```python
from build123d import *

# Parameters (mm, degrees)
ESBO_O2_W                                   = 14
ESBO_O2_H                                   = 46
RESSALTO_EXTRUS_O1_DEPTH                    = 6
CORTE_EXTRUS_O1_DEPTH                       = 49.456165758
FURO_DE_DI_METRO_7_5_7_5_1_D                = 7.5
CORTE_EXTRUS_O2_DEPTH                       = 49.456165758
ESBO_O10_W                                  = 5
ESBO_O10_H                                  = 4
RESSALTO_EXTRUS_O2_DEPTH                    = 5
BROCA_DE_ROSQUEAR_PARA_TARRAXA_DE_M31_D     = 2.5
BROCA_DE_ROSQUEAR_PARA_TARRAXA_DE_M31_DEPTH = 4
BROCA_DE_ROSQUEAR_PARA_TARRAXA_DE_M31_TIP   = 0.751075774
FURO_DE_DI_METRO_6_0_6_1_D                  = 6
CHANFRO1_SIZE                               = 1
FURO_DE_DI_METRO_3_0_3_1_D                  = 3
FURO_DE_DI_METRO_3_0_3_1_DEPTH              = 1
FURO_DE_DI_METRO_3_0_3_1_TIP                = 0.901290929
ESBO_O14_R                                  = 5.55
CORTE_EXTRUS_O4_DEPTH                       = 5


with BuildPart() as part:
    # Esboço2 → Ressalto-extrusão1 (new body)
    with BuildSketch(Plane(origin=(0, 0, 0), x_dir=(1, 0, 0), z_dir=(0, 1, 0))):
        with Locations((7, 23)):
            Rectangle(ESBO_O2_W, ESBO_O2_H)
    extrude(amount=RESSALTO_EXTRUS_O1_DEPTH)

    # Esboço6 → Corte-extrusão1 (cut, through all)
    with BuildSketch(Plane(origin=(0, 6, 0), x_dir=(1, 0, 0), z_dir=(0, 1, 0))):
        with BuildLine():
            Line((4.5, 46), (4.5, 31.538348415))
            ThreePointArc((4.5, 31.538348415), (1.233718703, 28.968626967), (0, 25))
            Line((0, 25), (0, 46))
            Line((0, 46), (4.5, 46))
        make_face()
        with BuildLine():
            Line((9.5, 46), (9.5, 31.538348415))
            ThreePointArc((9.5, 31.538348415), (12.766281297, 28.968626967), (14, 25))
            Line((14, 25), (14, 46))
            Line((14, 46), (9.5, 46))
        make_face()
    extrude(amount=-CORTE_EXTRUS_O1_DEPTH, mode=Mode.SUBTRACT)

    # Furo de diâmetro Ø7.5 (7.5)1 (through all)
    with Locations(Plane(origin=(7, 6, -13.5), x_dir=(0, 0, 1), z_dir=(0, 1, 0))):
        with Locations((0, 0)):
            Hole(FURO_DE_DI_METRO_7_5_7_5_1_D / 2)

    # Esboço9 → Corte-extrusão2 (cut, through all)
    with BuildSketch(Plane(origin=(0, 6, 0), x_dir=(1, 0, 0), z_dir=(0, 1, 0))):
        with BuildLine():
            Line((0, 13.5), (0, 0))
            Line((0, 0), (4.5, 0))
            Line((4.5, 0), (4.5, 6.961651585))
            ThreePointArc((4.5, 6.961651585), (1.233718703, 9.531373033), (0, 13.5))
        make_face()
        with BuildLine():
            Line((9.5, 0), (9.5, 6.961651585))
            ThreePointArc((9.5, 6.961651585), (12.766281297, 9.531373033), (14, 13.5))
            Line((14, 13.5), (14, 0))
            Line((14, 0), (9.5, 0))
        make_face()
    extrude(amount=-CORTE_EXTRUS_O2_DEPTH, mode=Mode.SUBTRACT)

    # Esboço10 → Ressalto-extrusão2 (add)
    with BuildSketch(Plane(origin=(0, 6, 0), x_dir=(1, 0, 0), z_dir=(0, 1, 0))):
        with Locations((7, 44)):
            Rectangle(ESBO_O10_W, ESBO_O10_H)
        with Locations((7, 2)):
            Rectangle(ESBO_O10_W, ESBO_O10_H)
    extrude(amount=RESSALTO_EXTRUS_O2_DEPTH)

    # Broca de rosquear para tarraxa de M31
    with Locations(Plane(origin=(7, 11, -2), x_dir=(0, 0, 1), z_dir=(0, 1, 0))):
        with Locations((0, 0), (-42, 0)):
            Hole(BROCA_DE_ROSQUEAR_PARA_TARRAXA_DE_M31_D / 2, depth=BROCA_DE_ROSQUEAR_PARA_TARRAXA_DE_M31_DEPTH)
            with Locations((0, 0, -(BROCA_DE_ROSQUEAR_PARA_TARRAXA_DE_M31_DEPTH + BROCA_DE_ROSQUEAR_PARA_TARRAXA_DE_M31_TIP / 2))):  # 118° drill point
                Cone(0, BROCA_DE_ROSQUEAR_PARA_TARRAXA_DE_M31_D / 2, BROCA_DE_ROSQUEAR_PARA_TARRAXA_DE_M31_TIP, mode=Mode.SUBTRACT)

    # Furo de diâmetro Ø6.0 (6)1 (through all)
    with Locations(Plane(origin=(7, 6, -25), x_dir=(0, 0, 1), z_dir=(0, 1, 0))):
        with Locations((0, 0)):
            Hole(FURO_DE_DI_METRO_6_0_6_1_D / 2)

    # Chanfro1
    chanfro1_edges = [part.edges().sort_by_distance(p)[0] for p in [
        (0, 0, -19.25),
        (7, 0, -46),
        (9.5, 5.5, -46),
        (12.766281297, 0, -28.968626967),
        (9.5, 0, -38.769174208),
        (4.5, 0, -38.769174208),
        (4.5, 5.5, -46),
        (1.233718703, 0, -28.968626967),
        (14, 0, -19.25),
        (7, 0, 0),
        (1.233718703, 0, -9.531373033),
        (4.5, 0, -3.480825792),
        (4.5, 5.5, 0),
        (9.5, 0, -3.480825792),
        (9.5, 5.5, 0),
        (12.766281297, 0, -9.531373033),
    ]]
    chamfer(chanfro1_edges, length=CHANFRO1_SIZE)

    # Furo de diâmetro Ø3.0 (3)1
    with Locations(Plane(origin=(7, 6, -36), x_dir=(0, 0, 1), z_dir=(0, 1, 0))):
        with Locations((0, 0)):
            Hole(FURO_DE_DI_METRO_3_0_3_1_D / 2, depth=FURO_DE_DI_METRO_3_0_3_1_DEPTH)
            with Locations((0, 0, -(FURO_DE_DI_METRO_3_0_3_1_DEPTH + FURO_DE_DI_METRO_3_0_3_1_TIP / 2))):  # 118° drill point
                Cone(0, FURO_DE_DI_METRO_3_0_3_1_D / 2, FURO_DE_DI_METRO_3_0_3_1_TIP, mode=Mode.SUBTRACT)

    # Esboço14 → Corte-extrusão4 (cut)
    with BuildSketch(Plane.XZ):
        with Locations(Location((7, -25, 0), (0, 0, 270))):
            Circle(ESBO_O14_R)
    extrude(amount=-CORTE_EXTRUS_O4_DEPTH, mode=Mode.SUBTRACT)


solid = part.part
```
The listing builds one solid part. Answer for the finished solid, in the listing's coordinates (mm). A direction names the side the tool comes from. Coordinates: 2 decimals unless noted, no trailing zeros. Loops run counter-clockwise (first coordinate to the right, second up) from the corner with the lowest first, then second, coordinate; pieces in that order, holes last. Notation, with made-up numbers: (56.5, 17) - (115.5, 17) arc R32 ccw to (115.5, 54) - close; hole circle Ø4 at (-3.75, 51). An arc over 180 degrees is marked (long way). Use a Markdown table: item, result. Add a question column.
1) For faces 1 (the flat face through (9.5, 5, -40)), 2 (the cylindrical face through (4.718, 2.958, -10.524)), 3 (the cylindrical face through (6.1, 5.5, -34.8)), 4 (the flat face through (5, 0.5, -38)), determine the directions among +Z, -Z, +X, -X, +Y, -Y from which every point of the face is accessible in a straight line to the end or side of a thin tool.
2) The part is cut by section B-B, the plane z = -41.5. Give the vertices of the cut face in (x, y), and give its area (3 significant figures).
3) Find the intervals of material crossed by line 1 (Z direction, x = 7, y = 9.5); line 2 (X direction, y = 8.75, z = -2); line 3 (Z direction, x = 9.75, y = 3.5), in increasing order.
4) Given pin 1 (5.5 mm diameter, centred on x = 8.5, z = -24, fed in from -Y); pin 2 (4 mm diameter, centred on x = 5, z = -22.5, fed in from +Y); pin 3 (3 mm diameter, centred on x = 2, y = 5.5, fed in from +Z); pin 4 (3.5 mm diameter, centred on x = 7, z = -25, fed in from -Y), each flat-ended and moving along its own axis, determine where each tip first touches the part or whether it passes through.
5) The mould has two halves that part along X. Classify faces 5 (the cylindrical face through (7.1, 5.5, -22)), 6 (the flat face through (8, 11, -43)), 7 (the flat face through (5, 6.1, -45.5)): released by +X, released by -X, zero draft, split by the parting line, or undercut.
6) The part is cut by section A-A, the plane y = 8.25. Give the vertices of the cut face in (x, z), and give its area (3 significant figures).
7) The part is cut by section C-C, the plane z = -20. Give the vertices of the cut face in (x, y).
Here are the results:
| question | item | result |
|---|---|---|
| 1 | face 1 | -Z, +X, +Y, -Y |
| 1 | face 2 | +Y, -Y |
| 1 | face 3 | +Y |
| 1 | face 4 | -Z, -X, -Y |
| 2 | outline | (4.5, 1) - (5.5, 0) - (8.5, 0) - (9.5, 1) - (9.5, 6) - (4.5, 6) - close |
| 2 | area | 29.0 mm^2 |
| 3 | line 1 | z = -46 to -45.25, -42.75 to -42, -4 to -3.25, -0.75 to 0 |
| 3 | line 2 | x = 4.5 to 5.75, 8.25 to 9.5 |
| 3 | line 3 | z = -31.44 to -29.82, -20.18 to -16.05, -10.95 to -7.06 |
| 4 | pin 1 | stops at y = 5 |
| 4 | pin 2 | stops at y = 6 |
| 4 | pin 3 | stops at z = -7.44 |
| 4 | pin 4 | passes through |
| 5 | face 5 | undercut |
| 5 | face 6 | zero draft |
| 5 | face 7 | released by -X |
| 6 | outline | (4.5, -45) - (5.5, -46) - (8.5, -46) - (9.5, -45) - (9.5, -42) - (4.5, -42) - close; (4.5, -4) - (9.5, -4) - (9.5, -1) - (8.5, 0) - (5.5, 0) - (4.5, -1) - close; hole circle Ø2.5 at (7, -44); hole circle Ø2.5 at (7, -2) |
| 6 | area | 28.2 mm^2 |
| 7 | outline | (0, 1) - (1, 0) - (4.59, 0) - (4.59, 5) - (9.41, 5) - (9.41, 0) - (13, 0) - (14, 1) - (14, 6) - (0, 6) - close |
